Source: CAD feature listing. Evaluate the final solid. Frame: model axes, mm. Face numbers are marked on the shaded views. A direction names the side the tool comes from. Round coordinates to 2 decimals unless told otherwise and drop trailing zeros. Order: outer loops, then holes, each group sorted by start corner. A loop starts at its lowest first (then second) coordinate and runs counter-clockwise, first axis right, second up. Notation, with made-up numbers: (52.5, 64.5) - (76.5, 64.5) arc R12 ccw to (76.5, 78.5) - close; hole circle Ø11 at (0, -28). An arc over 180 degrees is marked (long way). Put each result on its own line as item: value. Start each with the question number.
1) Section C-C on y = 41. Output: boundary loops of the cut face in (x, z), then the cut area to 3 significant figures.
2) Access query for the marked faces 1, 2 and 3. Directions: +Z, -Z, +X, -X, +Y, -Y. A direction counts if a zero-diameter tool reaches every point of the face in a straight line with its end or side. Return the directions, or none.
3) Section D-D on z = 46. Output: boundary loops of the cut face in (x, y), then the cut area to 3 significant figures.
4) Section A-A on y = 65. Output: boundary loops of the cut face in (x, z).
5) Contact query for flat-ended pins moving along their axis: P1, Ø8, axis at x = -6, y = 36.5, coming from the +Z side; P2, Ø6, axis at x = -16.5, z = 6, coming from the -Y side; P3, Ø8, axis at x = -8, y = 48, coming from the -Z side; P4, Ø11, axis at x = -7.5, z = 4.5, coming from the +Y side. Output: stop coordinate, or through.
6) Line query: probe 1 along X at (y, z) = (82, -2); probe 2 along Z at (x, y) = (-11.75, 80.5); probe 3 along Z at (x, y) = (-7.25, 71). Output: solid intervals per line, ascending. Write a range as [from, to].
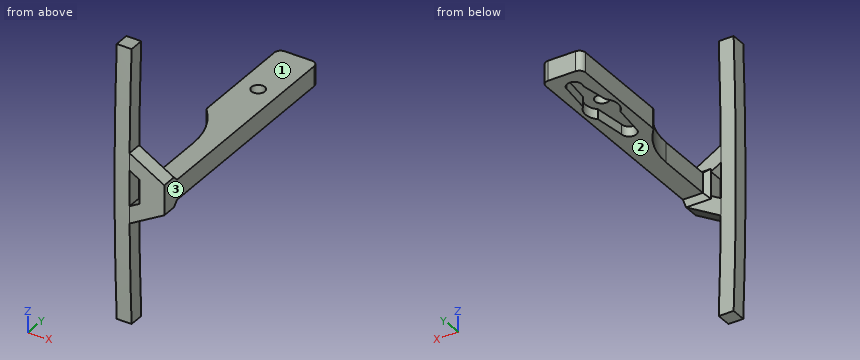
Autodesk Inventor part; units mm, degrees
ref_plane "YZ Plane" through (0, 0, 0) normal (1, 0, 0) x (0, 1, 0)
ref_plane "XZ Plane" through (0, 0, 0) normal (0, 1, 0) x (-1, 0, 0)
ref_plane "XY Plane" through (0, 0, 0) normal (0, 0, 1) x (1, 0, 0)
sketch "Skizze2" plane through (0, 0, 0) normal (0, 0, 1) x (1, 0, 0)
  line L0 (-45.7004, 0) -> (8.2208, 0)
  line L1 (0, -18.1036) -> (0, 108.6213)
  circle A0 centre (-8, 65) radius 2.7
  line L2 (0, 0) -> (0, 87.5)
  arc A1 (0, 87.5) -> (-2.5, 90) centre (-2.5, 87.5) ccw
  line L3 (-13.5, 90) -> (-2.5, 90)
  arc A2 (-13.5, 90) -> (-16, 87.5) centre (-13.5, 87.5) ccw
  line L4 (-16, 87.5) -> (-16, 45)
  line L5 (-8, 0) -> (-8, 25)
  line L6 (0, 0) -> (-8, 0)
  arc A3 (-8, 25) -> (-16, 45) centre (-37.9973, 24.6011) ccw
  point P0 (0, 0)
  point P1 (-4, 0)
  dimension "d0" = 90
  dimension "d1" = 8
  dimension "d2" = 16
  dimension "d4" = 2.5
  dimension "d5" = 2.5
  dimension "d6" = 5.4
  dimension "d8" = 25
  dimension "d11" = 25
  dimension "d16" = 2.5
  dimension "d17" = 2.5
  dimension "d18" = 2.5
  dimension "d19" = 2.5
  dimension "d90" = 45
  dimension "d126" = 30
  dimension "d131" = 40
  dimension "d132" = 8
extrude "Extrusion1" add sketch "Skizze2" along normal mid plane 8
sketch "Skizze5" plane through (-8, 0, 4) normal (0, -1, 0) x (1, 0, 0)
  line L0 (8, -8) -> (8, 0)
  line L1 (0, 0) -> (8, 0)
  line L2 (0, -8) -> (0, 0)
  line L3 (8, -8) -> (0, -8)
  line L4 (-2, -10) -> (-2, 2)
  line L5 (-2, 2) -> (10, 2)
  line L6 (10, 2) -> (10, -10)
  line L7 (10, -10) -> (-2, -10)
  line L8 (8, -10) -> (8, 2)
  line L9 (8, -10) -> (-6, -18.0829)
  line L10 (8, -10) -> (48, -10) construction
  line L11 (8, 2) -> (-6, 10.0829)
  line L12 (8, 2) -> (48, 2) construction
  line L13 (-6, 26.9678) -> (-6, -33.1167)
  line L14 (-2, 0.8453) -> (-6, 3.1547)
  line L15 (-6, -11.1547) -> (-2, -8.8453)
  point P0 (8, -4)
  dimension "d103" = 2
  dimension "d104" = 150
  dimension "d107" = 150
  dimension "d108" = 6
  dimension "d113" = 6
  dimension "d114" = 6
extrude "Extrusion3" add sketch "Skizze5" along normal blind 6 contours L3 L2 L1 L0 | L8 L7 L4 L5 L1 L2 L3 | L9 L13 L15 L4 L7 | L5 L4 L14 L13 L11
sketch "Skizze6" plane through (-14, 0, -14.0829) normal (-1, 0, 0) x (0, 0, 1)
  arc A0 (-91.4171, 6.8936) -> (119.5829, 6.8936) centre (14.0829, 1117.4186) ccw
  line L0 (14.0829, 1343.255) -> (14.0829, -237.5996)
  line L1 (-134.6641, 0) -> (162.8299, 0)
  line L2 (6.9282, 0) -> (0, 0)
  line L3 (0, 0) -> (0, -6)
  line L4 (6.9282, -6) -> (0, -6)
  line L5 (6.9282, 0) -> (6.9282, -6)
  line L6 (28.1658, 0) -> (21.2376, 0)
  line L7 (21.2376, 0) -> (21.2376, -6)
  line L8 (28.1658, -6) -> (21.2376, -6)
  line L9 (28.1658, 0) -> (28.1658, -6)
  line L10 (69.0829, 4.8846) -> (69.0829, -11.7632)
  line L11 (-40.9171, 6.8936) -> (-40.9171, -11.0991)
  arc A1 (-40.9171, 1.3407) -> (69.0829, 1.3407) centre (14.0829, 1117.4186) ccw
  arc A2 (-92.1649, -0.9783) -> (120.3307, -0.9783) centre (14.0829, 1117.4186) ccw
  point P0 (14.0829, 0)
  point P1 (-40.9171, 0.6181)
  point P2 (69.0829, -4.6666)
  point P3 (69.0829, 0.908)
  point P4 (-40.9171, 1.6575)
  point P5 (-40.9171, -4.6666)
  dimension "d122" = 6
  dimension "d127" = 110
extrude "Extrusion4" add sketch "Skizze6" along normal blind 6 contours A1 L1 L11 | L1 L3 A2 L11 | A1 L0 A2 L5 L1 | L10 L1 A1 | A1 L1 L7 A2 L0 | L1 L5 A2 L3 | L10 A2 L9 L1 | L1 L9 A2 L7
chamfer "Fasen6" distance 2 angle 45 3 edges at (-4, 0, -4) (-8, 0, 0) (-4, 0, 4)
fillet "Rundung1" radius 2 1 edges at (-16, 45, 0)
sketch "Skizze7" plane through (0, 0, -4) normal (0, 0, -1) x (-1, 0, 0)
  arc A0 (15.4998, 44.447) -> (16, 45.7701) centre (14, 45.7701) ccw
  line L0 (16, 45.7701) -> (16, 87.5)
  arc A1 (16, 87.5) -> (13.5, 90) centre (13.5, 87.5) ccw
  line L1 (13.5, 90) -> (2.5, 90)
  arc A2 (2.5, 90) -> (0, 87.5) centre (2.5, 87.5) ccw
  line L2 (0, 87.5) -> (0, 2)
  line L3 (8, 2) -> (0, 2)
  line L4 (8, 2) -> (8, 25)
  arc A3 (15.4998, 44.447) -> (8, 25) centre (37.9973, 24.6011) ccw
  circle A4 centre (8, 65) radius 2.7
  circle A5 centre (8, 65) radius 6.5
  line L5 (8, 85) -> (8, 45)
  line L6 (12.5, 82.2483) -> (12.5, 48.2483)
  line L7 (3.5, 48.5932) -> (3.5, 82.5932)
  circle A6 centre (8, 82) radius 3
  circle A7 centre (8, 48) radius 3
  line L8 (17.259, 81.9916) -> (-1.9844, 81.9916)
  line L9 (19.4429, 48.0084) -> (-6.0611, 48.0084)
  line L10 (5, 48.0084) -> (3.5, 60.3096)
  line L11 (11, 48.0084) -> (12.5, 60.3096)
  line L12 (3.5, 69.6904) -> (5, 81.9929)
  line L13 (12.5, 69.6904) -> (10.4193, 81.9916)
  point P0 (0, 0)
  point P1 (10.6543, 80.602)
  dimension "d142" = 6
  dimension "d133" = 13
  dimension "d136" = 20
  dimension "d137" = 20
  dimension "d143" = 3
  dimension "d144" = 6
  dimension "d145" = 3
  dimension "d146" = 9
extrude "Extrusion5" cut sketch "Skizze7" against normal blind 4 contours L9 L5 A7 | A7 L5 L9 | A7 L5 A5 L11 | A7 L10 A5 L5 | L5 L9 A7 | L5 A7 L9 | L6 A5 | A5 L5 A4 L6 | A5 L5 A6 L13 | L8 L5 A6 | A6 L13 L8 | A5 L7 L5 A4 | A5 L12 A6 L5 | A6 L5 L8 L13 | A5 L7 | A6 L8 L5 | L5 L8 A6
properties part number "Gripper neu"
Answer sheet:
1. outline: (-12.88, -4) - (0, -4) - (0, 4) - (-12.88, 4) - close
1. area: 103 mm^2
2. face 1: +Z, +X, -X, +Y
2. face 2: -Z, +X, -X, +Y
2. face 3: +Z, -Z, +X, +Y, -Y
3. outline: (-20, -5.07) - (-14, -5.07) - (-14, 0.93) - (-20, 0.93) - close
3. area: 36.0 mm^2
4. outline: (-16, -4) - (-14.5, -4) - (-14.5, 0) - (-10.7, 0) - (-10.7, 4) - (-16, 4) - close; (-5.3, 0) - (-1.5, 0) - (-1.5, -4) - (0, -4) - (0, 4) - (-5.3, 4) - close
5. P1: z = 4
5. P2: y = -6.01
5. P3: z = -4
5. P4: y = 90
6. probe 1: [-16, -11], [-5, 0]
6. probe 2: [-4, 4]
6. probe 3: [0, 4]
